Part print with two shaded views. Sizes in mm from the minimum x, y, z corner. A direction names the side the tool comes from. Give positions to 0.01 mm unless a question says otherwise; leave off trailing zeros. Order: outer loops, then holes, each group sorted by start corner. A loop starts at its lowest first (then second) coordinate and runs counter-clockwise, first axis right, second up. Notation, with made-up numbers: M -27.5,18.5 L -1.5,18.5 A22 cw -1.5,24.5 Z; hole C 19,5.5 d3. An arc over 180 degrees is marked long. Return JSON: item names as keys, results as strings.
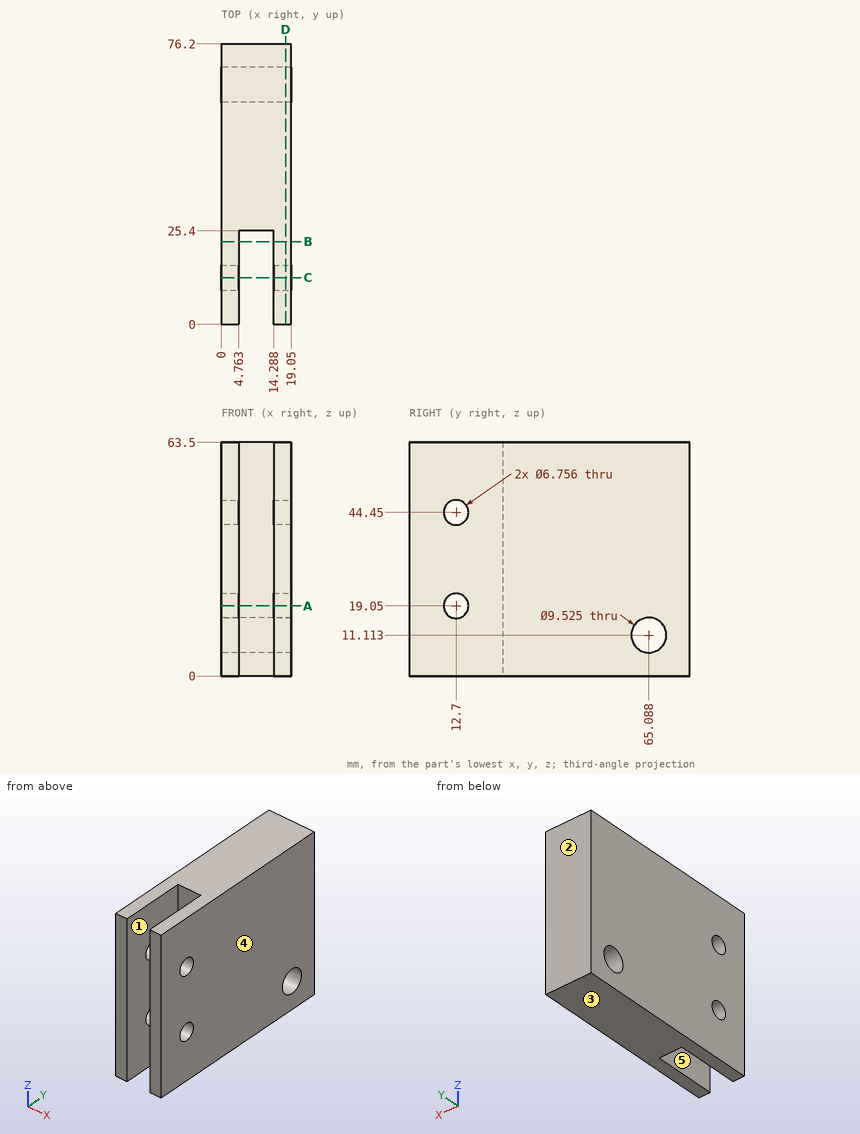
Q1. Band-saw the part on C-C (y = 12.7). Give the cut face in (x, z).
Established:
{"outline": "M 0,0 L 4.76,0 L 4.76,15.67 L 0,15.67 Z; M 0,22.43 L 4.76,22.43 L 4.76,41.07 L 0,41.07 Z; M 0,47.83 L 4.76,47.83 L 4.76,63.5 L 0,63.5 Z; M 14.29,0 L 19.05,0 L 19.05,15.67 L 14.29,15.67 Z; M 14.29,22.43 L 19.05,22.43 L 19.05,41.07 L 14.29,41.07 Z; M 14.29,47.83 L 19.05,47.83 L 19.05,63.5 L 14.29,63.5 Z"}
Q2. 3-axis set-ups, long thin cutter, end or side, ignore diameter. For the marked faces 1 and 2: which of +Z, -Z, +X, -X, +Y, -Y reach the whole face in a straight line?
Established:
{"face 1": "+Z, -Z, -Y", "face 2": "+Z, -Z, +X, -X, +Y"}
Q3. Band-saw the part on B-B (y = 22.5). Give the cut face in (x, z), then the cut area to 3 significant figures.
Established:
{"outline": "M 0,0 L 4.76,0 L 4.76,63.5 L 0,63.5 Z; M 14.29,0 L 19.05,0 L 19.05,63.5 L 14.29,63.5 Z", "area": "605 mm²"}
Q4. Band-saw the part on D-D (x = 17.5). Give the number of separate pieces and of enclosed holes in the cut face, then the cut area to 3 significant figures.
Established:
{"separate pieces": "1", "enclosed holes": "3", "area": "4,700 mm²"}
Q5. Pin check, flat tip, straight feed: pin 1 (5.5 mm diameter, centred on y = 12.7, z = 19.05, fed in from -X). Stop position of the tip, or through.
Established:
{"pin 1": "passes through"}
Q6. Probe line 1 along X through (y, z) = (13.5, 26); line 2 along Y through (x, z) = (17.3, 19.05); line 3 along Z through (x, y) = (2, 14.5). List the from-to ranges inside material, lowest first.
Established:
{"line 1": "x = 0 to 4.76, 14.29 to 19.05", "line 2": "y = 0 to 9.32, 16.08 to 76.2", "line 3": "z = 0 to 16.19, 21.91 to 41.59, 47.31 to 63.5"}
Q7. Band-saw the part on A-A (z = 19.05). Give the cut face in (x, y).
Established:
{"outline": "M 0,0 L 4.76,0 L 4.76,9.32 L 0,9.32 Z; M 0,16.08 L 4.76,16.08 L 4.76,25.4 L 14.29,25.4 L 14.29,16.08 L 19.05,16.08 L 19.05,76.2 L 0,76.2 Z; M 14.29,0 L 19.05,0 L 19.05,9.32 L 14.29,9.32 Z"}
Q8. Two-plate mould, pull along X, no slides. Class the marked faces 3, 4 and 5: +X half, -X half, draft (parallel to the pull), parting line (faces both ways), or undercut.
Established:
{"face 3": "draft", "face 4": "+X half", "face 5": "undercut"}
